CAD build for the part. Positions are in the model's coordinates, mm. Give positions to 0.01 mm unless a question says otherwise; leave off trailing zeros. Loops run counter-clockwise (first coordinate to the right, second up) from the corner with the lowest first, then second, coordinate; pieces in that order, holes last. Notation, with made-up numbers: M 55,36.25 L 111,36.25 A25 ccw 111,60.25 Z; hole C 86,-16.5 d1. An arc over 180 degrees is marked long. One line per question, with ' | ' between items.
```python
from build123d import *

# Parameters (mm, degrees)
SKETCH_1_R      = 1.6
SKETCH_1_W      = 105
SKETCH_1_H      = 48
EXTRUDE_1_DEPTH = 2
FILLET_1_R      = 3


with BuildPart() as part:
    # ｽｹｯﾁ1 → ﾎﾞｽ - 押し出し1 (new body)
    with BuildSketch(Plane.XY):
        with BuildLine():
            Line((-116.941733701, 29), (116.941733701, 29))
            ThreePointArc((116.941733701, 29), (121.697016283, 25.545084972), (119.880659963, 19.954915028))
            Line((119.880659963, 19.954915028), (52.5, -29))
            Line((52.5, -29), (-52.5, -29))
            Line((-52.5, -29), (-119.880659963, 19.954915028))
            ThreePointArc((-119.880659963, 19.954915028), (-121.697016283, 25.545084972), (-116.941733701, 29))
        make_face()
        with Locations((118.411196832, 21.977457514)):
            Circle(SKETCH_1_R, mode=Mode.SUBTRACT)
        with Locations((77.960347113, -7.411805101)):
            Circle(SKETCH_1_R, mode=Mode.SUBTRACT)
        with Locations(Location((-118.411196832, 21.977457514, 0), (0, 0, 180))):
            Circle(SKETCH_1_R, mode=Mode.SUBTRACT)
        with Locations(Location((-77.960347113, -7.411805101, 0), (0, 0, 180))):
            Circle(SKETCH_1_R, mode=Mode.SUBTRACT)
        Rectangle(SKETCH_1_W, SKETCH_1_H, mode=Mode.SUBTRACT)
        with BuildLine():
            Line((-57.5, 21), (-57.5, -13.299115956))
            ThreePointArc((-57.5, -13.299115956), (-59.138028501, -15.972135529), (-62.263355757, -15.726166939))
            Line((-62.263355757, -15.726166939), (-116.941733701, 24))
            Line((-116.941733701, 24), (-60.5, 24))
            ThreePointArc((-60.5, 24), (-58.378679656, 23.121320344), (-57.5, 21))
        make_face(mode=Mode.SUBTRACT)
        with BuildLine():
            Line((62.263355757, -15.726166939), (116.941733701, 24))
            Line((116.941733701, 24), (60.5, 24))
            ThreePointArc((60.5, 24), (58.378679656, 23.121320344), (57.5, 21))
            Line((57.5, 21), (57.5, -13.299115956))
            ThreePointArc((57.5, -13.299115956), (59.138028501, -15.972135529), (62.263355757, -15.726166939))
        make_face(mode=Mode.SUBTRACT)
    extrude(amount=EXTRUDE_1_DEPTH)

    # ﾌｨﾚｯﾄ1
    fillet_1_edges = [part.edges().sort_by_distance(p)[0] for p in [
        (-52.5, -29, 1),
        (-52.5, 24, 1),
        (-52.5, -24, 1),
        (52.5, -24, 1),
        (52.5, 24, 1),
        (116.941733701, 24, 1),
        (-116.941733701, 24, 1),
    ]]
    fillet(fillet_1_edges, radius=FILLET_1_R)


solid = part.part
```
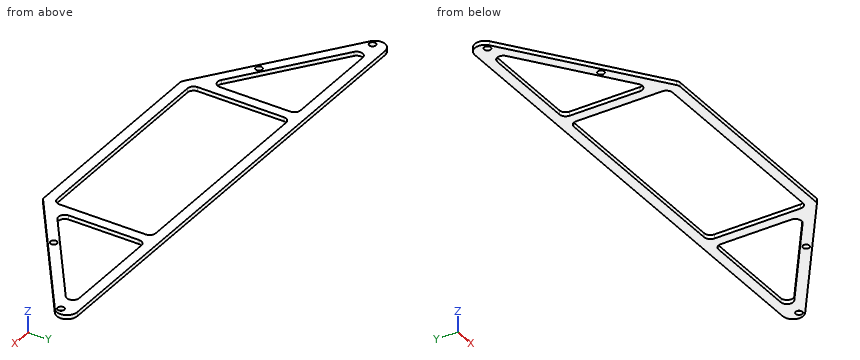
Item 1: Saw through at D-D on x = -105.5. Give the cut face in (y, z), and give its area (3 significant figures).
Conclusion:
outline: M 9.51,0 L 15.69,0 L 15.69,2 L 9.51,2 Z; M 24,0 L 29,0 L 29,2 L 24,2 Z | area: 22.4 mm²
Item 2: Drill centre lines: line 1 along Y through (x, z) = (-4.5, 1.7); line 2 along Y through (x, z) = (77.5, 1.5); line 3 along X through (y, z) = (1.5, 1.45). Where is each one in solid material? Low to high. Write a range as [from, to].
Conclusion:
line 1: [-29, -24], [24, 29] | line 2: [-10.84, -8.94], [-5.88, -4.66], [24, 29] | line 3: [-94.48, -85.97], [-57.5, -52.5], [52.5, 57.5], [85.97, 94.48]
Item 3: Saw through at A-A on x = -47. Give the cut face in (y, z), and give its area (3 significant figures).
Conclusion:
outline: M -29,0 L -24,0 L -24,2 L -29,2 Z; M 24,0 L 29,0 L 29,2 L 24,2 Z | area: 20.0 mm²
Item 4: Drop flat-ended pins along their axis: P1, Ø3.5, axis at x = -77.96, y = -7.41, coming from the +Z side; P2, Ø0.6, axis at y = -9.5, z = 1, coming from the -X side; P3, Ø0.6, axis at x = 95.5, z = 0.5, coming from the -Y side. Give the stop position or say it passes through.
Conclusion:
P1: z = 2 | P2: x = -79.75 | P3: y = 2.02
Item 5: Saw through at C-C on z = 0.3. State how many separate pieces and enclosed holes the cut face has, and give its area (3 significant figures).
Conclusion:
separate pieces: 1 | enclosed holes: 7 | area: 3,050 mm²
Item 6: Saw through at B-B on y = 2.5. Give the cut face in (x, z).
Conclusion:
outline: M -95.86,0 L -87.35,0 L -87.35,2 L -95.86,2 Z; M -57.5,0 L -52.5,0 L -52.5,2 L -57.5,2 Z; M 52.5,0 L 57.5,0 L 57.5,2 L 52.5,2 Z; M 87.35,0 L 95.86,0 L 95.86,2 L 87.35,2 Z
